```python
from build123d import *

# Parameters (mm, degrees)
SKETCH_W     = 27
SKETCH_H     = 40
PAD_DEPTH    = 1
SKETCH001_R  = 0.5
PAD001_DEPTH = 4


with BuildPart() as part:
    # Sketch → Pad (new body)
    with BuildSketch(Plane.XY):
        with Locations((-13.5, 20)):
            Rectangle(SKETCH_W, SKETCH_H)
    extrude(amount=PAD_DEPTH)

    # Sketch001 (on Face4 of Pad) → Pad001 (join)
    with BuildSketch(Plane(origin=(-27, 0, 0), x_dir=(0, -1, 0), z_dir=(-1, 0, 0))):
        with Locations((-39.5, 0.5)):
            Circle(SKETCH001_R)
    extrude(amount=PAD001_DEPTH)

    # Mirrored: part across YZ


with BuildPart() as part_1:
    add(part.part)
    add(part.part.mirror(Plane.YZ))


solid = part_1.part
```
Input: part model. Units: mm. Frame: model coordinates. Give positions to 0.01 mm unless a question says otherwise; leave off trailing zeros. Order: outer loops, then holes, each group sorted by start corner. A loop starts at its lowest first (then second) coordinate and runs counter-clockwise, first axis right, second up. Notation, with made-up numbers: M 53,-4 L 106,-4 A15 ccw 106,9 Z; hole C 58.5,69 d7. An arc over 180 degrees is marked long. One line per question, with ' | ' between items. Start each with the question number.
1. First-contact query: pin 1 Ø0.5 at (y, z) = (28, 0.5) entering from -X. Flat tip, straight axial feed; report the tip coordinate or a pass-through.
2. Material intervals for probe 1 along X at (y, z) = (10, 0.95); probe 2 along Y at (x, z) = (28, 0.8), sorted ascending. Write a range as [from, to].
3. Section query A-A (z = 0.8). Return the cut outline in (x, y).
4. Section query B-B (y = 37.5). Return the cut outline in (x, z).
Here are the results:
1) pin 1: x = -27
2) probe 1: [-27, 27] | probe 2: [39.1, 39.9]
3) outline: M -31,39.1 L -27,39.1 L -27,0 L 27,0 L 27,39.1 L 31,39.1 L 31,39.9 L 27,39.9 L 27,40 L -27,40 L -27,39.9 L -31,39.9 Z
4) outline: M -27,0 L 27,0 L 27,1 L -27,1 Z
